CAD build for the part. Positions are in the model's coordinates, mm. A direction names the side the tool comes from. Round coordinates to 2 decimals unless told otherwise and drop trailing zeros. Loops run counter-clockwise (first coordinate to the right, second up) from the corner with the lowest first, then second, coordinate; pieces in that order, holes last. Notation, with made-up numbers: (89, 76.25) -> (139, 76.25) arc R14 ccw to (139, 80.25) -> close; hole circle Ø5 at (89.5, 60.5). An arc over 180 degrees is marked (long way). Answer as CSV lines item,"result".
```python
from build123d import *

# Parameters (mm, degrees)
SKETCH001_W = 40
SKETCH001_H = 25
SKETCH001_R = 1.75
PAD_DEPTH   = 20


with BuildPart() as part:
    # Sketch001 → Pad (new body)
    with BuildSketch(Plane.XY.offset(5)):
        Rectangle(SKETCH001_W, SKETCH001_H)
        with Locations((-1.746173, -8.246033)):
            Circle(SKETCH001_R, mode=Mode.SUBTRACT)
        with Locations((1.752117, 8.249296)):
            Circle(SKETCH001_R, mode=Mode.SUBTRACT)
        with Locations((15.75151, -8.249899)):
            Circle(SKETCH001_R, mode=Mode.SUBTRACT)
        with Locations((-15.749744, 8.249736)):
            Circle(SKETCH001_R, mode=Mode.SUBTRACT)
        Polygon((3.75, -4), (3.75, 4), (-3.75, 4), (-3.75, 2.5), (2, 2.5), (2, -2.5), (-3.75, -2.5), (-3.75, -4), align=None, mode=Mode.SUBTRACT)
    extrude(amount=PAD_DEPTH)


solid = part.part
```
Q1. Slice it at A-A, the plane y = 0.75. Give the cut face in (x, z).
Results:
outline,"(-20, 5) -> (2, 5) -> (2, 25) -> (-20, 25) -> close; (3.75, 5) -> (20, 5) -> (20, 25) -> (3.75, 25) -> close"
Q2. Two-plate mould, pull along Y, no slides. Class faces 3 (the flat face through (0, 12.5, 15)), 4 (the cylindrical face through (17.37, -8.92, 14.86)), 5 (the flat face through (-3.75, 3, 15)), 6 (the flat face through (0, 0, 25)): pulls with the +Y half, pulls with the -Y half, needs draft (parallel to the pull), parting line crosses it, or undercut.
Results:
face 3,"pulls with the +Y half"
face 4,"undercut"
face 5,"undercut"
face 6,"needs draft"
Q3. Slice it at C-C, the plane z = 8.25. Give the cut face in (x, y).
Results:
outline,"(-20, -12.5) -> (20, -12.5) -> (20, 12.5) -> (-20, 12.5) -> close; hole circle Ø3.5 at (-15.75, 8.25); hole (-3.75, -4) -> (3.75, -4) -> (3.75, 4) -> (-3.75, 4) -> (-3.75, 2.5) -> (2, 2.5) -> (2, -2.5) -> (-3.75, -2.5) -> close; hole circle Ø3.5 at (-1.75, -8.25); hole circle Ø3.5 at (1.75, 8.25); hole circle Ø3.5 at (15.75, -8.25)"
Q4. Tool access for faces 1 (the flat face through (-1, 2.5, 15)), 2 (the flat face through (20, 0, 15)): list every direction of +Z, -Z, +X, -X, +Y, -Y with a clear straight run to the whole face (end or side of a thin tool).
Results:
face 1,"+Z, -Z"
face 2,"+Z, -Z, +X, +Y, -Y"
Q5. Slice it at D-D, the plane y = -9.5. Give the cut face in (x, z), and give its area (3 significant figures).
Results:
outline,"(-20, 5) -> (-2.97, 5) -> (-2.97, 25) -> (-20, 25) -> close; (-0.53, 5) -> (14.53, 5) -> (14.53, 25) -> (-0.53, 25) -> close; (16.98, 5) -> (20, 5) -> (20, 25) -> (16.98, 25) -> close"
area,"702 mm2"
Q6. Probe L1, parallel to X at y = -8.25, z = 7.5; L2, parallel to X at y = -3.25, z = 7.25; L3, parallel to X at y = -2.25, z = 20. List the from-to ranges inside material, lowest first. Write a range as [from, to].
Results:
L1,"[-20, -3.5], [0, 14], [17.5, 20]"
L2,"[-20, -3.75], [3.75, 20]"
L3,"[-20, 2], [3.75, 20]"
Q7. Slice it at B-B, the plane x = 15.5. Give the cut face in (y, z).
Results:
outline,"(-12.5, 5) -> (-9.98, 5) -> (-9.98, 25) -> (-12.5, 25) -> close; (-6.52, 5) -> (12.5, 5) -> (12.5, 25) -> (-6.52, 25) -> close"
